For this review, take the finished solid that the model builds, in its own axes (mm). Face numbers are marked on the shaded views. A direction names the side the tool comes from. Coordinates: 2 decimals unless noted, no trailing zeros. Order: outer loops, then holes, each group sorted by start corner. A loop starts at its lowest first (then second) coordinate and runs counter-clockwise, first axis right, second up. Notation, with made-up numbers: (-21.5, 34.25) -> (32.5, 34.25) arc R21 ccw to (32.5, 52.25) -> close; hole circle Ø9 at (31.25, 52.25). An arc over 180 degrees is marked (long way). Write item = value, one per line. Start each with the question number.
1) Machinability: for the marked faces 4 and 5, which of the approach directions +Z, -Z, +X, -X, +Y, -Y give a long, thin tool a straight path to every point of the face, cutting with its end or side? Answer none if there is none.
2) Insertion check: pin 1 Ø8 at (x, z) = (9.5, -8.5) entering from -Y; pin 2 Ø5 at (y, z) = (-22.86, -13.2) entering from -X; pin 3 Ø1.5 at (x, y) = (-9, 19.5) entering from +Z; pin 4 Ø10 at (x, z) = (-2, -11.5) entering from -Y. Each pin has a flat end and moves straight along its axis. Give the tip position at first contact, or say it passes through.
3) Consider section C-C on x = 0. Give the boundary of the cut face in (y, z), and give its area (3 significant figures).
4) Draft analysis for pull direction Y (two halves, no side actions). For the marked faces 1, 2 and 3, state which applies: +Y half, -Y half, draft (parallel to the pull), parting line (faces both ways), or undercut.
5) Consider section B-B on y = 0. State how many separate pieces and enclosed holes the cut face has, and give its area (3 significant figures).
6) Wall thickness on probe 1 along Y at (x, z) = (3, 0); probe 2 along X at (y, z) = (17, 22); probe 3 along Y at (x, z) = (-12.1, -13.2): over which ranges is each line inside the solid? List them lowest first. Write a range as [from, to].
7) Consider section A-A on z = 0. Give the boundary of the cut face in (x, y).
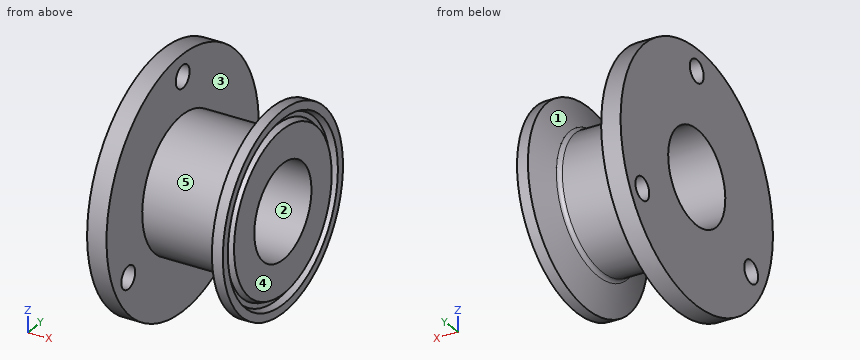
from build123d import *

# Parameters (mm, degrees)
M5_CLEARANCE_HOLE1_REACH  = 59.107
M5_CLEARANCE_HOLE1_BORE_R = 2.9
SKETCH5_R                 = 42
SKETCH5_R_2               = 32
CUT_EXTRUDE_THIN1_DEPTH   = 55.572226802


with BuildPart() as part:
    # Sketch1 → Revolve1 (revolve)
    with BuildSketch(Plane.XY, mode=Mode.PRIVATE) as revolve1_sk:
        with BuildLine():
            Line((-15.404727216, 12), (-15.404727216, 34))
            Line((-15.404727216, 34), (-10.404727216, 34))
            Line((-10.404727216, 34), (-10.404727216, 17))
            Line((-10.404727216, 17), (8.794935567, 17))
            ThreePointArc((8.794935567, 17), (9.450533434, 17.206709213), (9.869004233, 17.752070976))
            Line((9.869004233, 17.752070976), (12.598027216, 25.25))
            Line((12.598027216, 25.25), (15.404727216, 25.25))
            Line((15.404727216, 25.25), (15.404727216, 23.1186))
            Line((15.404727216, 23.1186), (13.829927216, 22.450137059))
            Line((13.829927216, 22.450137059), (13.829927216, 21.187062941))
            Line((13.829927216, 21.187062941), (15.404727216, 20.5186))
            Line((15.404727216, 20.5186), (15.404727216, 12))
            Line((15.404727216, 12), (-15.404727216, 12))
        make_face()
    revolve(revolve1_sk.sketch.rotate(Axis((0, 0, 0), (1, 0, 0)), 90), axis=Axis((0, 0, 0), (1, 0, 0)))

    # M5 Clearance Hole1 bore → M5 Clearance Hole1 (cut, up to next)
    with BuildSketch(Plane.ZY.offset(15.404727216), mode=Mode.PRIVATE) as m5_clearance_hole1_sk1:
        with Locations((-13.199999999, -22.86307066)):
            Circle(M5_CLEARANCE_HOLE1_BORE_R)
    m5_clearance_hole1_tool1 = extrude(m5_clearance_hole1_sk1.sketch, amount=-M5_CLEARANCE_HOLE1_REACH, mode=Mode.PRIVATE) & part.part
    # M5 Clearance Hole1 bore → M5 Clearance Hole1 (cut, up to next)
    with BuildSketch(Plane.ZY.offset(15.404727216), mode=Mode.PRIVATE) as m5_clearance_hole1_sk2:
        with Locations((-13.200000001, 22.863070659)):
            Circle(M5_CLEARANCE_HOLE1_BORE_R)
    m5_clearance_hole1_tool2 = extrude(m5_clearance_hole1_sk2.sketch, amount=-M5_CLEARANCE_HOLE1_REACH, mode=Mode.PRIVATE) & part.part
    # M5 Clearance Hole1 bore → M5 Clearance Hole1 (cut, up to next)
    with BuildSketch(Plane.ZY.offset(15.404727216), mode=Mode.PRIVATE) as m5_clearance_hole1_sk3:
        with Locations((26.4, 1e-09)):
            Circle(M5_CLEARANCE_HOLE1_BORE_R)
    m5_clearance_hole1_tool3 = extrude(m5_clearance_hole1_sk3.sketch, amount=-M5_CLEARANCE_HOLE1_REACH, mode=Mode.PRIVATE) & part.part
    add(m5_clearance_hole1_tool1.solids().sort_by_distance((-15.404727, -22.863071, -13.2))[0], mode=Mode.SUBTRACT)
    add(m5_clearance_hole1_tool2.solids().sort_by_distance((-15.404727, 22.863071, -13.2))[0], mode=Mode.SUBTRACT)
    add(m5_clearance_hole1_tool3.solids().sort_by_distance((-15.404727, 0, 26.4))[0], mode=Mode.SUBTRACT)

    # Sketch5 → Cut-Extrude-Thin1 (cut, through all)
    with BuildSketch(Plane(origin=(-10.404727216, 0, 0), x_dir=(0, 0, -1), z_dir=(1, 0, 0))):
        Circle(SKETCH5_R)
        Circle(SKETCH5_R_2, mode=Mode.SUBTRACT)
    extrude(amount=-CUT_EXTRUDE_THIN1_DEPTH, mode=Mode.SUBTRACT)


solid = part.part
Answer sheet:
q1.face_4 = +Z, -Z, +X, +Y, -Y
q1.face_5 = none
q2.pin_1 = -24.53
q2.pin_2 = 12.11
q2.pin_3 = through
q2.pin_4 = -15.71
q3.outline = circle Ø34 at (0, 0); hole circle Ø24 at (0, 0)
q3.area = 456 mm2
q4.face_1 = parting line
q4.face_2 = undercut
q4.face_3 = draft
q5.separate_pieces = 3
q5.enclosed_holes = 0
q5.area = 494 mm2
q6.probe_1 = [-17, -12], [12, 17]
q6.probe_2 = [-15.4, -10.4]
q6.probe_3 = [-29.15, -25.76], [-19.96, 19.96], [25.76, 29.15]
q7.outline = (-15.4, -32) -> (-10.4, -32) -> (-10.4, -17) -> (8.79, -17) arc R1.14 cw to (9.87, -17.75) -> (12.6, -25.25) -> (15.4, -25.25) -> (15.4, -23.12) -> (13.83, -22.45) -> (13.83, -21.19) -> (15.4, -20.52) -> (15.4, -12) -> (-15.4, -12) -> close; (-15.4, 12) -> (15.4, 12) -> (15.4, 20.52) -> (13.83, 21.19) -> (13.83, 22.45) -> (15.4, 23.12) -> (15.4, 25.25) -> (12.6, 25.25) -> (9.87, 17.75) arc R1.14 cw to (8.79, 17) -> (-10.4, 17) -> (-10.4, 32) -> (-15.4, 32) -> close
